Source: three-view drawing plus pictorial views. Frame: mm from the lowest corner of the part. Give positions to 0.01 mm unless a question says otherwise; leave off trailing zeros. Order: outer loops, then holes, each group sorted by start corner. A loop starts at its lowest first (then second) coordinate and runs counter-clockwise, first axis right, second up. Notation, with made-up numbers: (12.5, -3) -> (28.5, -3) arc R7 cw to (28.5, 9) -> close; hole circle Ø7 at (48.5, 49). An arc over 180 degrees is marked (long way). One line per question, with ' | ' between items.
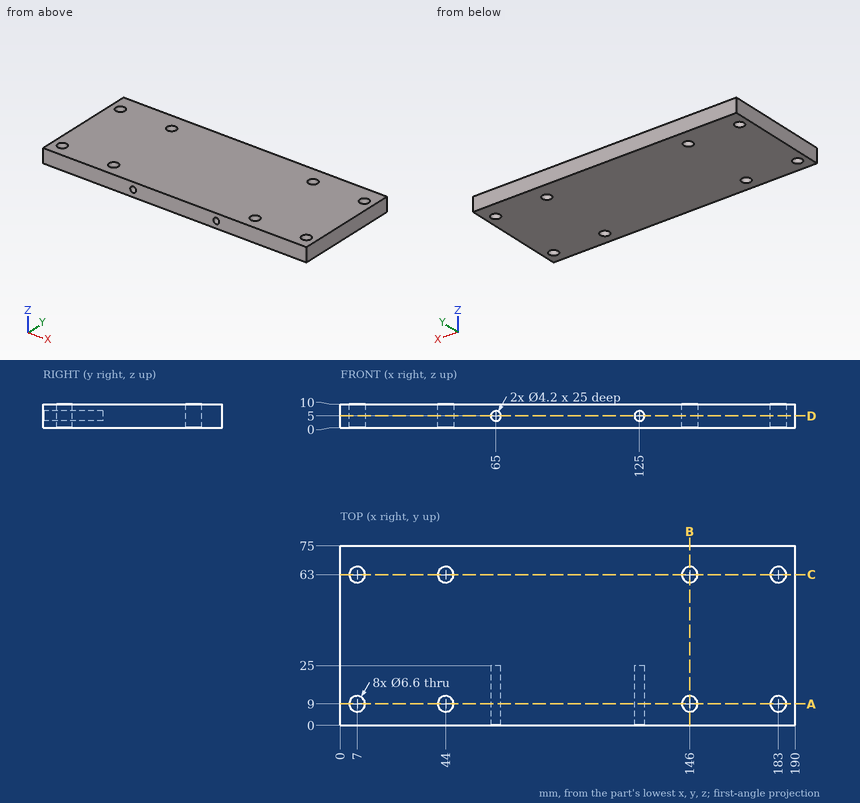
1) Section B-B on x = 146. Return loops of the section in (y, z).
Check result:
outline: (0, 0) -> (5.7, 0) -> (5.7, 10) -> (0, 10) -> close; (12.3, 0) -> (59.7, 0) -> (59.7, 10) -> (12.3, 10) -> close; (66.3, 0) -> (75, 0) -> (75, 10) -> (66.3, 10) -> close
2) Section A-A on y = 9. Return loops of the section in (x, z), plus the area to 3 significant figures.
Check result:
outline: (0, 0) -> (3.7, 0) -> (3.7, 10) -> (0, 10) -> close; (10.3, 0) -> (40.7, 0) -> (40.7, 10) -> (10.3, 10) -> close; (47.3, 0) -> (142.7, 0) -> (142.7, 10) -> (47.3, 10) -> close; (149.3, 0) -> (179.7, 0) -> (179.7, 10) -> (149.3, 10) -> close; (186.3, 0) -> (190, 0) -> (190, 10) -> (186.3, 10) -> close; hole circle Ø4.2 at (65, 5); hole circle Ø4.2 at (125, 5) | area: 1,610 mm^2
3) Section D-D on z = 5. Count the separate pieces of the cut face and the enclosed holes in it, plus the area to 3 significant figures.
Check result:
separate pieces: 1 | enclosed holes: 8 | area: 13,800 mm^2
4) Material intervals for probe 1 along Y at (x, z) = (7, 2.75); probe 2 along Z at (x, y) = (65, 16.75); probe 3 along Y at (x, z) = (180, 2.5), sorted ascending. Write a range as from..to.
Check result:
probe 1: y = 0..5.7, 12.3..59.7, 66.3..75 | probe 2: z = 0..2.9, 7.1..10 | probe 3: y = 0..7.63, 10.37..61.63, 64.37..75
5) Contact query for a flat-ended pin moving along its axis: pin 1 Ø4 at (x, z) = (125, 5) entering from -Y. Output: stop coordinate, or through.
Check result:
pin 1: stops at y = 25
6) Section C-C on y = 63. Return loops of the section in (x, z).
Check result:
outline: (0, 0) -> (3.7, 0) -> (3.7, 10) -> (0, 10) -> close; (10.3, 0) -> (40.7, 0) -> (40.7, 10) -> (10.3, 10) -> close; (47.3, 0) -> (142.7, 0) -> (142.7, 10) -> (47.3, 10) -> close; (149.3, 0) -> (179.7, 0) -> (179.7, 10) -> (149.3, 10) -> close; (186.3, 0) -> (190, 0) -> (190, 10) -> (186.3, 10) -> close
